Can you work these out from the model? Positions are in its coordinate system, mm. Coordinates: 2 decimals unless noted, no trailing zeros. Order: outer loops, then holes, each group sorted by start corner. A loop starts at its lowest first (then second) coordinate and runs counter-clockwise, first axis right, second up. Notation, with made-up numbers: (-12, -31.5) -> (17, -31.5) arc R4 ccw to (17, -27.5) -> close; hole circle Ø4 at (56.25, 55). An arc over 180 degrees is marked (long way). Return JSON: item names as keys, results as strings. Group by question number.
1) If we section it at C-C, the plane x = 6.46: Please give me the cut outline in (y, z).
2) If we section it at A-A, the plane z = 3.25: Please give me the cut outline in (x, y).
3) If I drill on probe 1 along X at (y, z) = (18, 1.85); probe 2 along X at (y, z) = (25, 3.1); probe 3 along Y at (x, z) = (-46.5, 3.05), over which ranges is the centre line in solid material (lowest first)? Write a range as from..to.
4) For pin 1 (1.5 mm diameter, centred on y = 40.5, z = 3.5, fed in from +X); pin 2 (0.7 mm diameter, centred on x = 2, z = 2.5, fed in from +Y), each with a flat end and sliding along its axis, tell me the tip position at first contact or that it passes through.
5) If we section it at B-B, the plane y = 16: Please give me the cut outline in (x, z), then the cut area to 3 significant figures.
from build123d import *

# Parameters (mm, degrees)
F1_DEPTH = 5


with BuildPart() as f1:
    # F0 (on Top) → F1 (new body)
    with BuildSketch(Plane.XY):
        with BuildLine():
            Line((0, 28.5), (0, 50))
            Line((0, 50), (-50, 50))
            Line((-50, 50), (-50, 28.5))
            ThreePointArc((-50, 28.5), (-49.56066, 27.43934), (-48.5, 27))
            Line((-48.5, 27), (-47.876976, 27))
            ThreePointArc((-47.876976, 27), (-47.198184, 27.162375), (-46.66635, 27.614345))
            ThreePointArc((-46.66635, 27.614345), (-43.079484, 29.236499), (-39.839877, 27))
            ThreePointArc((-39.839877, 27), (-39.448681, 24.960662), (-40.132594, 23))
            ThreePointArc((-40.132594, 23), (-43.132912, 21.264252), (-46.362337, 22.523436))
            ThreePointArc((-46.362337, 22.523436), (-46.86111, 22.87571), (-47.458959, 23))
            Line((-47.458959, 23), (-48.5, 23))
            ThreePointArc((-48.5, 23), (-49.56066, 22.56066), (-50, 21.5))
            Line((-50, 21.5), (-50, 0))
            Line((-50, 0), (0, 0))
            Line((0, 0), (0, 21.5))
            ThreePointArc((0, 21.5), (0.43934, 22.56066), (1.5, 23))
            Line((1.5, 23), (2.346308, 23))
            ThreePointArc((2.346308, 23), (2.961343, 22.868113), (3.468224, 22.495643))
            ThreePointArc((3.468224, 22.495643), (6.775996, 21.163191), (9.832615, 23))
            ThreePointArc((9.832615, 23), (8.755451, 28.426496), (3.287213, 27.586552))
            ThreePointArc((3.287213, 27.586552), (2.760678, 27.154606), (2.097418, 27))
            Line((2.097418, 27), (1.5, 27))
            ThreePointArc((1.5, 27), (0.43934, 27.43934), (0, 28.5))
        make_face()
    extrude(amount=F1_DEPTH)


solid = f1.part
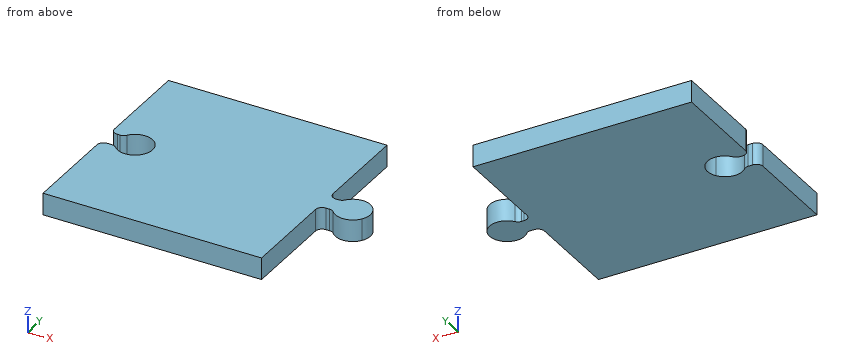
Result sheet:
{
 "1": {"outline": "(21.15, 0) -> (29.15, 0) -> (29.15, 5) -> (21.15, 5) -> close"},
 "2": {"outline": "(-50, 0) -> (0, 0) -> (0, 21.5) arc R1.5 cw to (1.5, 23) -> (2.35, 23) arc R1.5 cw to (3.47, 22.5) arc R4 ccw (long way) to (3.29, 27.59) arc R1.5 cw to (2.1, 27) -> (1.5, 27) arc R1.5 cw to (0, 28.5) -> (0, 50) -> (-50, 50) -> (-50, 28.5) arc R1.5 ccw to (-48.5, 27) -> (-47.88, 27) arc R1.5 ccw to (-46.67, 27.61) arc R4 cw to (-39.84, 27) arc R4 cw to (-40.13, 23) arc R4 cw to (-46.36, 22.52) arc R1.5 ccw to (-47.46, 23) -> (-48.5, 23) arc R1.5 ccw to (-50, 21.5) -> close"},
 "3": {"probe 1": "x = -50..0", "probe 2": "x = -39.45..10.46", "probe 3": "y = 0..22.65, 27.83..50"},
 "4": {"pin 1": "stops at x = 0", "pin 2": "stops at y = 27.02"},
 "5": {"outline": "(-50, 0) -> (0, 0) -> (0, 5) -> (-50, 5) -> close", "area": "250 mm2"}
}
